Study the drawing (mm; zero at the part's minimum x, y, z) and answer. A direction names the side the tool comes from. Give positions to 0.01 mm unless a question says otherwise; leave off trailing zeros. Write each loop counter-clockwise with the first axis right and the second up, starting at its lowest first coordinate (ties: lowest second). Pieces come first, ordered by that corner, then holes. Notation, with made-up numbers: (9.5, 16) - (54.5, 16) arc R16 ccw to (54.5, 22) - close; hole circle Ø9 at (-18, -24.75). An arc over 180 degrees is marked (long way). Answer as CSV lines item,"result".
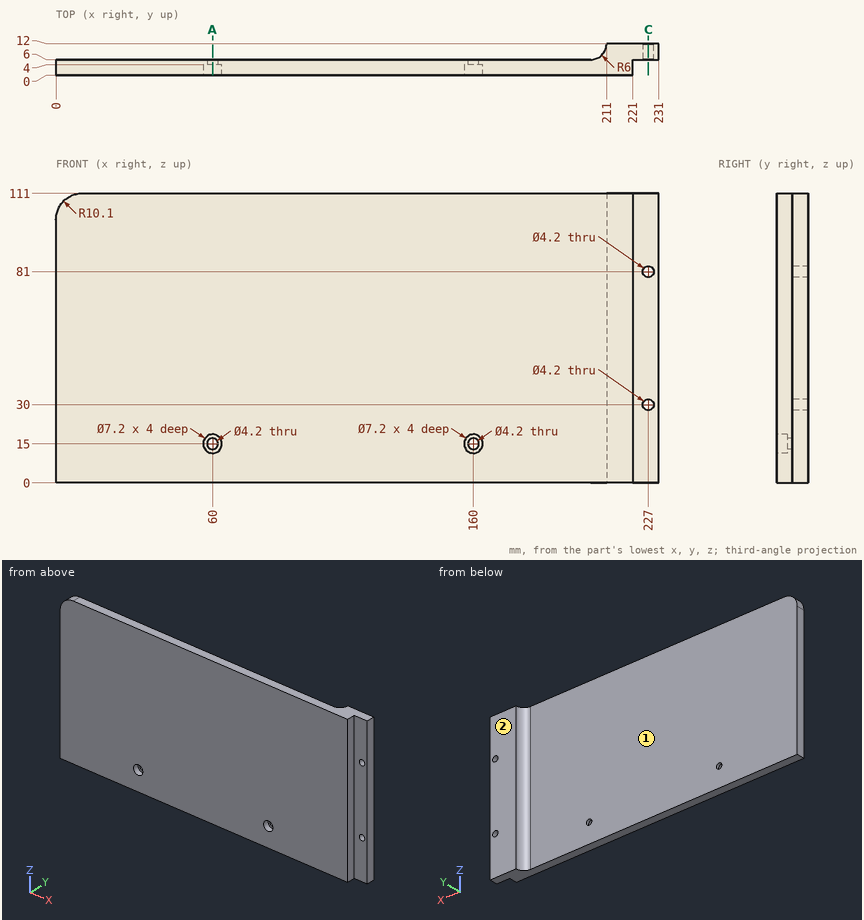
(1) Find the intervals of material crossed by L1, parallel to Z at x = 227, y = 7.45; L2, parallel to X at y = 3.75, z = 18; L3, parallel to Z at x = 60, y = 5.45, in increasing order.
Worked out:
L1,"z = 0 to 27.9, 32.1 to 78.9, 83.1 to 111"
L2,"x = 0 to 58.01, 61.99 to 158.01, 161.99 to 221"
L3,"z = 0 to 12.9, 17.1 to 111"
(2) For the marked faces 1 and 2, determine the directions among +Z, -Z, +X, -X, +Y, -Y from which every point of the face is accessible in a straight line to the end or side of a thin tool.
Worked out:
face 1,"+Z, -Z, -X, +Y"
face 2,"+Z, -Z, +X, -X, +Y"
(3) A cutting plane is placed at C-C (x = 227). Write down the section's boundary in (y, z).
Worked out:
outline,"(6, 0) - (12, 0) - (12, 27.9) - (6, 27.9) - close; (6, 32.1) - (12, 32.1) - (12, 78.9) - (6, 78.9) - close; (6, 83.1) - (12, 83.1) - (12, 111) - (6, 111) - close"
(4) A cutting plane is placed at A-A (x = 60). Write down the section's boundary in (y, z), and give its area (3 significant figures).
Worked out:
outline,"(0, 0) - (6, 0) - (6, 12.9) - (4, 12.9) - (4, 11.4) - (0, 11.4) - close; (0, 18.6) - (4, 18.6) - (4, 17.1) - (6, 17.1) - (6, 111) - (0, 111) - close"
area,"629 mm^2"
(5) Each of these flat-tipped pins is pushed along its axis until it touches: P1, Ø10, axis at x = 154, z = 66.5, coming from the +Y side; P2, Ø2.5, axis at x = 227, z = 81, coming from the -Y side; P3, Ø3, axis at y = 4, z = 37, coming from the +X side; P4, Ø2, axis at x = 61.5, z = 16, coming from the -Y side. Where does it stop, or does it pass through?
Worked out:
P1,"stops at y = 6"
P2,"passes through"
P3,"stops at x = 221"
P4,"stops at y = 4"
